Part model, mm, in its own coordinate system. Face numbers are marked on the shaded views. Give positions to 0.01 mm unless a question says otherwise; leave off trailing zeros. Loops run counter-clockwise (first coordinate to the right, second up) from the corner with the lowest first, then second, coordinate; pieces in that order, holes last. Notation, with made-up numbers: M -22.5,24 L 36.5,24 A16 ccw 36.5,35 Z; hole C 63,73.25 d4. An arc over 180 degrees is marked long. Put each result on its own line as item: value. Start each with the question number.
```python
from build123d import *

# Parameters (mm, degrees)
F0_W     = 76
F0_H     = 130
F1_DEPTH = 63
F2_SIZE2 = 25
F2_SIZE  = 20
F3_R     = 2
F4_DEPTH = 125.2523570347
F5_R     = 8.5
F6_DEPTH = 76.001
F7_W     = 38
F7_H     = 31.5
F8_DEPTH = 38


with BuildPart() as f1:
    # F0 (on Top) → F1 (new body)
    with BuildSketch(Plane.XY):
        Rectangle(F0_W, F0_H)
    extrude(amount=F1_DEPTH)

    # F2
    f2_edges = [f1.edges().sort_by_distance(p)[0] for p in [
        (0, 65, 0),
    ]]
    f2_side = f1.faces().sort_by_distance((0, 0, 0))[0]
    chamfer(f2_edges, length=F2_SIZE, length2=F2_SIZE2, reference=f2_side)

    # F3 (on face) → F4 (cut, through all)
    with BuildSketch(Plane(origin=(0, 27.4390243902, -21.9512195122), x_dir=(-1, 0, 0), z_dir=(0, 0.7808688094, -0.6246950476))):
        with Locations((0, 44.1190877335)):
            Circle(F3_R)
    extrude(amount=-F4_DEPTH, mode=Mode.SUBTRACT)

    # F5 (on face) → F6 (cut, through all)
    with BuildSketch(Plane.YZ.offset(38)):
        with Locations((3, 15)):
            Circle(F5_R)
    extrude(amount=-F6_DEPTH, mode=Mode.SUBTRACT)

    # F7 (on face) → F8 (join)
    with BuildSketch(Plane.XZ.offset(65)):
        with Locations((0, 47.25)):
            Rectangle(F7_W, F7_H)
    extrude(amount=F8_DEPTH)


solid = f1.part
```
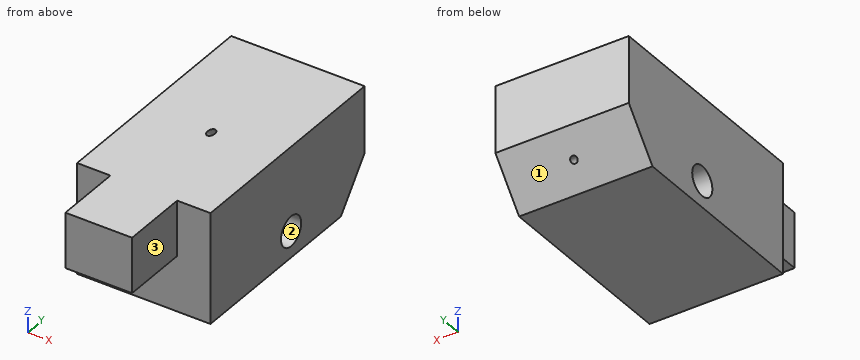
1) Band-saw the part on D-D on x = 21. Give the cut face in (y, z), then the cut area to 3 significant figures.
2) Wall check: L1, parallel to Z at x = 15, y = 3; L2, parallel to X at y = -87.5, z = 34; L3, parallel to Y at x = 25.5, z = 25.5. Give the ranges that are in metal, low to high.
3) Band-saw the part on A-A on x = -5.5. Give the cut face in (y, z).
4) Band-saw the part on B-B on y = 3. State how many separate pieces and enclosed holes the cut face has, then the cut area to 3 significant figures.
5) Pin check, flat tips, straight feed: pin 1 Ø19.5 at (y, z) = (3, 15) entering from -X; pin 2 Ø16 at (y, z) = (-81.5, 47) entering from +X; pin 3 Ø3 at (x, z) = (17, 13.5) entering from -Y; pin 4 Ø16 at (y, z) = (-81.5, 52.5) entering from -X. Stop position of each tip, or through.
6) Mould opens along Y. For the marked faces 1, 2 and 3 say: +Y half, -Y half, draft (parallel to the pull), parting line (faces both ways), or undercut.
Evaluation:
1. outline: M -65,0 L 45,0 L 65,25 L 65,63 L -65,63 Z; hole C 3,15 d17
1. area: 7,710 mm2
2. L1: 0 to 6.5, 23.5 to 63
2. L2: -19 to 19
2. L3: -65 to 65
3. outline: M -103,31.5 L -65,31.5 L -65,0 L 45,0 L 65,25 L 65,63 L -103,63 Z; hole C 3,15 d17
4. separate pieces: 2
4. enclosed holes: 1
4. area: 3,480 mm2
5. pin 1: x = -38
5. pin 2: x = 19
5. pin 3: y = -65
5. pin 4: x = -19
6. face 1: +Y half
6. face 2: undercut
6. face 3: draft
